The figure shows three views and two pictorial views of one solid part (mm, origin at its lowest corner). Answer the questions. Coordinates: 2 decimals unless noted, no trailing zeros. Write each loop counter-clockwise with the first axis right and the second up, starting at its lowest first coordinate (ties: lowest second). Pieces come first, ordered by that corner, then holes.
Item 1: Section C-C (x = 5.5) is taken. Give the vertices of the cut face in (y, z), then the cut area to 4 significant figures.
Item 2: Section B-B (y = 1.6) is taken. Give the vertices of the cut face in (x, z), then the cut area to 4 significant figures.
Item 3: Section A-A (z = 82) is taken. Give the vertices of the cut face in (x, y).
Item 4: Straight lines are drawn through the part: probe 1 along Z at (x, y) = (16.5, 0.2); probe 2 along X at (y, z) = (0.7, 87); probe 3 along Z at (x, y) = (3, 0.7). For each, find the intervals that lie inside material, in ascending order.
Item 5: Each of these flat-tipped pins is pushed along its axis until it touches: P1, Ø1.2, axis at x = 16.5, y = 1, coming from the +Z side; P2, Ø1.2, axis at y = 1, z = 96.5, coming from the -X side; P3, Ø0.8, axis at y = 1, z = 96.5, coming from the +X side. Where does it stop, or does it pass through?
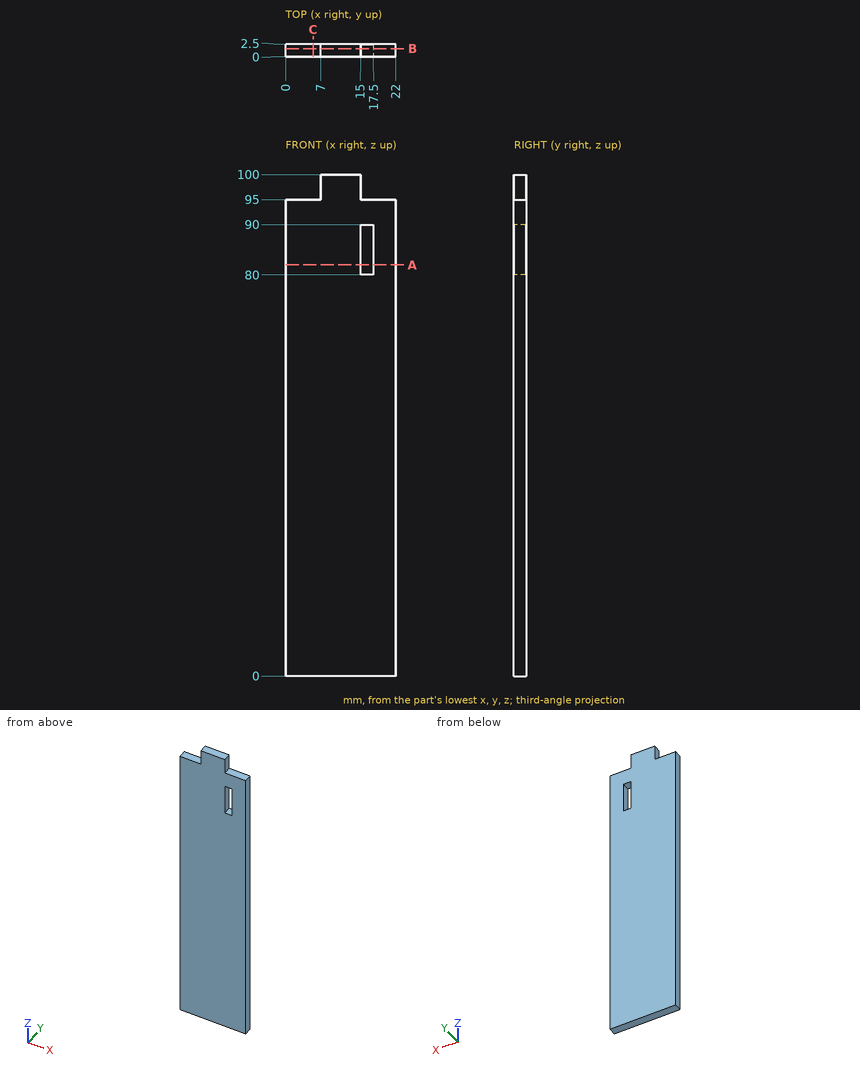
Established:
1. outline: (0, 0) - (2.5, 0) - (2.5, 95) - (0, 95) - close
1. area: 237.5 mm2
2. outline: (0, 0) - (22, 0) - (22, 95) - (15, 95) - (15, 100) - (7, 100) - (7, 95) - (0, 95) - close; hole (15, 80) - (17.5, 80) - (17.5, 90) - (15, 90) - close
2. area: 2,105 mm2
3. outline: (0, 0) - (15, 0) - (15, 2.5) - (0, 2.5) - close; (17.5, 0) - (22, 0) - (22, 2.5) - (17.5, 2.5) - close
4. probe 1: z = 0 to 80, 90 to 95
4. probe 2: x = 0 to 15, 17.5 to 22
4. probe 3: z = 0 to 95
5. P1: stops at z = 95
5. P2: stops at x = 7
5. P3: stops at x = 15
